Autodesk Inventor part; units mm, degrees
ref_plane "Work Plane1" through (0, 0, -32.5) normal (0, 0, -1) x (-1, 0, 0)
ref_plane "Work Plane2" through (0, 0, 0) normal (0, -1, 0) x (1, 0, 0)
ref_plane "YZ Plane" through (0, 0, 0) normal (1, 0, 0) x (0, 1, 0)
sketch "Sketch1" plane through (0, 0, 0) normal (0, 1, 0) x (-1, 0, 0)
  circle A0 centre (0, 0) radius 32.5
  dimension "d0" = 65
extrude "Extrusion1" add sketch "Sketch1" along normal blind 38.5
sketch "Sketch2" plane through (0, 0, 0) normal (0, -1, 0) x (1, 0, 0)
  circle A0 centre (0, 0) radius 25.5
  dimension "d3" = 51
extrude "Extrusion2" add sketch "Sketch2" along normal blind 23.4
chamfer "Chamfer1" distance 3 angle 45 2 edges at (32.5, 38.5, 0) (32.5, 0, 0)
sketch "Sketch3" plane through (0, -23.4, 0) normal (0, -1, 0) x (1, 0, 0)
  line L0 (0, 0) -> (0, -10.5) construction
  circle A0 centre (0, 0) radius 25.5
  line L1 (0, -10.5) -> (5.75, -10.5)
  line L2 (5.75, -10.5) -> (5.75, -24.8433)
  line L3 (0, -10.5) -> (-5.75, -10.5)
  line L4 (-5.75, -10.5) -> (-5.75, -24.8433)
  line L5 (5.75, -24.8433) -> (-5.75, -24.8433)
  line L6 (-15, 15) -> (15, 15) construction
  line L7 (15, 15) -> (15, -15) construction
  line L8 (15, -15) -> (-15, -15) construction
  line L9 (-15, -15) -> (-15, 15) construction
  line L10 (-15, 15) -> (15, -15) construction
  line L11 (15, 15) -> (-15, -15) construction
  line L12 (5.65, 5.65) -> (-5.65, 5.65) construction
  line L13 (-5.65, 5.65) -> (-5.65, -5.65) construction
  line L14 (-5.65, -5.65) -> (5.65, -5.65) construction
  line L15 (5.65, -5.65) -> (5.65, 5.65) construction
  line L16 (5.65, 5.65) -> (-5.65, -5.65) construction
  line L17 (-5.65, 5.65) -> (5.65, -5.65) construction
  dimension "d10" = 10.5
  dimension "d14" = 5.75
  dimension "d15" = 5.75
  dimension "d16" = 30
  dimension "d17" = 30
  dimension "d35" = 11.3
  dimension "d36" = 11.3
hole "Hole1" at (15, -23.4, -15) at (-15, -23.4, -15) at (15, -23.4, 15) at (-15, -23.4, 15) direction (0, 1, 0) diameter 2.5 depth 4
thread "Thread1"
thread "Thread2"
thread "Thread3"
thread "Thread4"
extrude "Extrusion3" cut sketch "Sketch3" against normal blind 12 contours L5 A0 | L4 L3 L1 L2 L5
hole "Hole2" at (5.65, -23.4, 5.65) at (5.65, -23.4, -5.65) at (-5.65, -23.4, 5.65) at (-5.65, -23.4, -5.65) direction (0, 1, 0) diameter 2.1 depth 3 tip angle 118
thread "Thread5"
thread "Thread6"
thread "Thread7"
thread "Thread8"
ref_plane "Work Plane1" through (0, 0, -32.5) normal (0, 0, -1) x (-1, 0, 0)
sketch "Sketch4" plane through (0, 0, -32.5) normal (0, 0, -1) x (-1, 0, 0)
  line L0 (-25.5, -23.4) -> (25.5, -23.4)
  line L1 (-32.5, 3) -> (32.5, 3)
  line L2 (32.5, 35.5) -> (-32.5, 35.5)
  line L3 (0, -23.4) -> (0, 18.1) construction
  line L4 (32.5, 3) -> (32.5, 35.5)
  line L5 (-32.5, 3) -> (-32.5, 35.5)
  line L6 (-32.5, 17.6) -> (32.5, 17.6)
  line L7 (32.5, 17.6) -> (32.5, 18.6)
  line L8 (32.5, 18.6) -> (-32.5, 18.6)
  line L9 (-32.5, 18.6) -> (-32.5, 17.6)
  line L10 (-32.5, 17.6) -> (32.5, 18.6) construction
  line L11 (32.5, 17.6) -> (-32.5, 18.6) construction
  line L12 (-20, 18.1) -> (20, 18.1) construction
  line L13 (-20, 9.1) -> (20, 9.1)
  line L14 (20, 27.1) -> (-20, 27.1)
  arc A0 (-20, 27.1) -> (-20, 9.1) centre (-20, 18.1) ccw
  arc A1 (20, 9.1) -> (20, 27.1) centre (20, 18.1) ccw
  line L15 (0, 18.1) -> (-15, 18.1)
  line L16 (0, 18.1) -> (15, 18.1)
  circle A2 centre (-15, 18.1) radius 6.35
  circle A3 centre (15, 18.1) radius 6.35
  line L17 (-20, 25.6) -> (20, 25.6)
  arc A4 (20, 10.6) -> (20, 25.6) centre (20, 18.1) ccw
  line L18 (20, 10.6) -> (-20, 10.6)
  arc A5 (-20, 25.6) -> (-20, 10.6) centre (-20, 18.1) ccw
  point P0 (0, 0)
  point P1 (-5.75, -23.4)
  point P2 (5.75, -23.4)
  dimension "d52" = 41.5
  dimension "d53" = 1
  dimension "d54" = 20
  dimension "d55" = 18
  dimension "d56" = 15
  dimension "d57" = 15
  dimension "d58" = 12.7
  dimension "d59" = 12.7
  dimension "d64" = 1.5
extrude "Extrusion5" cut sketch "Sketch4" against normal blind 15 contours A2 L8 L6 | L6 A2 | A3 L6 | L6 A3 L8 | A2 L8 | L8 A3
sketch "Sketch5" plane through (0, 0, 0) normal (1, 0, 0) x (0, 1, 0)
  line L0 (3, -32.5) -> (35.5, -32.5)
  line L1 (18.6, -33) -> (17.6, -33)
  line L2 (17.6, -33) -> (17.6, -32)
  line L3 (17.6, -32) -> (18.6, -32)
  line L4 (18.6, -32) -> (18.6, -33)
  line L5 (18.6, -33) -> (17.6, -32) construction
  line L6 (17.6, -33) -> (18.6, -32) construction
  line L7 (-35.78, 0) -> (50.88, 0)
  point P0 (0, 0)
  point P1 (18.1, -32.5)
  point P2 (18.1, -32.5)
  point P3 (18.1, -32.5)
  dimension "d67" = 1
  dimension "d68" = 1
revolve "Revolution1" cut sketch "Sketch5" angle 360 about axis through (0, -10, 0) along (0, 1, 0)
ref_plane "Work Plane2" through (0, 0, 0) normal (0, -1, 0) x (1, 0, 0)
split "Split1" plane through (0, 0, 0) removes the side toward (0, 1, 0)
sketch "Sketch6" plane through (0, 0, 0) normal (0, 1, 0) x (1, 0, 0)
  point P0 (0, 0)
properties part number "SweepV0.991_BASE_Rev.1" material "LCP Plastic"
Work out the finished part from the listing and answer in its coordinate system (mm). A direction names the side the tool comes from. Give positions to 0.01 mm unless a question says otherwise; leave off trailing zeros. Loops run counter-clockwise (first coordinate to the right, second up) from the corner with the lowest first, then second, coordinate; pieces in that order, holes last. Notation, with made-up numbers: (25, 4.25) -> (52, 4.25) arc R8 ccw to (52, 14.25) -> close; hole circle Ø6 at (-34, 54). An arc over 180 degrees is marked (long way). Write item = value, one per line. Start each with the question number.
(1) The mould has two halves that part along X. Classify faces 1 (the flat face through (0, 0, 0)), 2 (the cylindrical face through (-5.5, -11.5, 24.9)), 3 (the cylindrical face through (-15.845, -21.372, 15.921)), 4 (the flat face through (-15, -19.4, -15)): +X half, -X half, draft (parallel to the pull), parting line (faces both ways), or undercut.
(2) Given pin 1 Ø5 at (x, z) = (-20, -3) entering from +Y; pin 2 Ø4 at (x, y) = (-18, -19.5) entering from -Z; pin 3 Ø3 at (x, y) = (-6.5, -4.5) entering from +Z (3 decimals); pin 4 Ø0.8 at (x, z) = (-15, 15.5) entering from -Y, each flat-ended and moving along its own axis, determine where each tip first touches the part or whether it passes through.
(3) Which of the six approach directions +Z, -Z, +X, -X, +Y, -Y give full straight-line access (tool end or side, diameter ignored) to faces 5 (the cylindrical face through (13.76, -21.37, 15.16)), 6 (the flat face through (0, -23.4, 1)), 7 (the flat face through (0, -17, -10.5))?
(4) Find section D-D on z = -20.5. Give the vertices of the cut face in (x, y), and give its area (3 significant figures).
(5) Find section A-A on z = -15. Give the vertices of the cut face in (x, y), and give its area (3 significant figures).
(6) Find section C-C on x = 20. Give the vertices of the cut face in (y, z).
(7) Find the intervals of material crossed by probe 1 along Z at (x, y) = (5.65, -22.3); probe 2 along X at (y, z) = (-21.3, 15); probe 3 along X at (y, z) = (-22.2, 5.65), in increasing order. Write a range as from..to.
(8) Find section B-B on y = -3.5. Give the vertices of the cut face in (x, z), and give its area (3 significant figures).
From the geometry:
q1.face_1 = draft
q1.face_2 = parting line
q1.face_3 = undercut
q1.face_4 = undercut
q2.pin_1 = 0
q2.pin_2 = -19.86
q2.pin_3 = 25.005
q2.pin_4 = -19.4
q3.face_5 = -Y
q3.face_6 = +Z, -Z, +X, -X, -Y
q3.face_7 = -Z, -Y
q4.outline = (-15.17, -23.4) -> (-5.75, -23.4) -> (-5.75, -11.4) -> (5.75, -11.4) -> (5.75, -23.4) -> (15.17, -23.4) -> (15.17, 0) -> (-15.17, 0) -> close
q4.area = 572 mm^2
q5.outline = (-20.62, -23.4) -> (-16.25, -23.4) -> (-16.25, -19.4) -> (-13.75, -19.4) -> (-13.75, -23.4) -> (-5.75, -23.4) -> (-5.75, -11.4) -> (5.75, -11.4) -> (5.75, -23.4) -> (13.75, -23.4) -> (13.75, -19.4) -> (16.25, -19.4) -> (16.25, -23.4) -> (20.62, -23.4) -> (20.62, 0) -> (-20.62, 0) -> close
q5.area = 807 mm^2
q6.outline = (-23.4, -15.82) -> (0, -15.82) -> (0, 15.82) -> (-23.4, 15.82) -> close
q7.probe_1 = -10.5..-6.7, -4.6..4.6, 6.7..24.87
q7.probe_2 = -20.62..-16.25, -13.75..13.75, 16.25..20.62
q7.probe_3 = -24.87..-6.7, -4.6..4.6, 6.7..24.87
q8.outline = circle Ø51 at (0, 0)
q8.area = 2,040 mm^2
